Geometry check sheet. Reference: the model listing, model coordinates, mm. A direction names the side the tool comes from. Coordinates: 2 decimals unless noted, no trailing zeros. Write each loop counter-clockwise with the first axis right and the second up, starting at its lowest first coordinate (ties: lowest second). Pieces come first, ordered by that corner, then holes. Notation, with made-up numbers: (-6, 19) -> (13, 19) arc R16 ccw to (13, 41) -> close; hole circle Ø6 at (35, -7). An arc over 180 degrees is marked (long way). Use a Markdown table: item, result.
```python
from build123d import *

# Parameters (mm, degrees)
F1_DEPTH       = 60
F3_D           = 5
F3_CSINK_D     = 7.7
F3_CSINK_ANGLE = 90
F5_DEPTH       = 29.6009997154
F6_W           = 50
F6_H           = 17.8652722283
F7_W           = 50
F7_H           = 17.6054795285
F8_DEPTH       = 5


with BuildPart() as f1:
    # F0 (on Front) → F1 (new body)
    with BuildSketch(Plane.XZ):
        Polygon((-88.3284620883, 15.3996990994), (-88.3284620883, 13.399699384), (-73.3284620883, 13.399699384), (-72.7784620883, 40.999699384), (-13.5784620883, 40.999699384), (-13.0284620883, 13.399699384), (1.9715379117, 13.399699384), (1.9715379117, 15.3996990994), (-11.0679203725, 15.3996990994), (-11.6179203725, 42.9996990994), (-74.7390038042, 42.9996990994), (-75.2890038042, 15.3996990994), align=None)
    extrude(amount=F1_DEPTH)

    # F3 (through all)
    with Locations(Plane.XY.offset(15.3996990994)):
        with Locations((-81.8087329462, -10), (-81.8087329462, -50), (-4.5481912304, -50), (-4.5481912304, -10)):
            CounterSinkHole(F3_D / 2, F3_CSINK_D / 2, counter_sink_angle=F3_CSINK_ANGLE)

    # F4 (on face) → F5 (cut, through all)
    with BuildSketch(Plane.XY.offset(42.9996990994)):
        Polygon((-48.3518556123, -30), (-69.7390038042, -10), (-69.7390038042, -50), align=None)
        Polygon((-21.6179203725, -5), (-64.7390038042, -5), (-43.1784620883, -25.1621474003), align=None)
        Polygon((-16.6179203725, -50), (-16.6179203725, -10), (-38.0050685644, -30), align=None)
        Polygon((-43.1784620883, -34.8378525997), (-64.7390038042, -55), (-21.6179203725, -55), align=None)
    extrude(amount=-F5_DEPTH, mode=Mode.SUBTRACT)

    # F6 (on face) + F7 (on face) → F8 (cut, symmetric)
    with BuildSketch(Plane(origin=(-10.756770725, 0, -0.2143559384), x_dir=(0, 1, 0), z_dir=(0.9998015058, 0, 0.0199235807))):
        with Locations((-30, 29.2899983673)):
            Rectangle(F6_W, F6_H)
    with BuildSketch(Plane(origin=(-75.565874151, 0, 1.505841695), x_dir=(0, -1, 0), z_dir=(-0.9998015058, 0, 0.0199235807))):
        with Locations((30, 27.6993555667)):
            Rectangle(F7_W, F7_H)
    extrude(amount=F8_DEPTH, both=True, dir=(0.9998015058, 0, 0.0199235807), mode=Mode.SUBTRACT)


solid = f1.part
```
Item 1: Depth check by flat-ended pin: P1, Ø6.5, axis at x = -81.81, y = -50, coming from the +Z side; P2, Ø12, axis at y = -12, z = 25, coming from the -X side; P3, Ø1, axis at y = -37, z = 42.5, coming from the -X side. Enter the tip coordinate at first touch or a pass-through.
Answer block:
| item | result |
|---|---|
| P1 | stops at z = 14.8 |
| P2 | stops at x = -75.22 |
| P3 | stops at x = -74.76 |
Item 2: Section check A-A on z = 25. Record the boundary of the cut face in (x, y), then the cut area to 3 significant figures.
Answer block:
| item | result |
|---|---|
| outline | (-75.1, -60) -> (-73.1, -60) -> (-73.1, -55) -> (-75.1, -55) -> close; (-75.1, -5) -> (-73.1, -5) -> (-73.1, 0) -> (-75.1, 0) -> close; (-13.26, -60) -> (-11.26, -60) -> (-11.26, -55) -> (-13.26, -55) -> close; (-13.26, -5) -> (-11.26, -5) -> (-11.26, 0) -> (-13.26, 0) -> close |
| area | 40.0 mm^2 |
Item 3: Tool access check on faces 5 (the flat face through (-32.549, -15.222, 42.014)), 6 (the flat face through (-46.7, -60, 41.4)). Record the directions out of +Z, -Z, +X, -X, +Y, -Y that give a thin tool (end or side, any length) a straight path to the whole face; none if there is none.
Answer block:
| item | result |
|---|---|
| face 5 | +Z, -Z |
| face 6 | +Z, -Z, +X, -X, -Y |
Item 4: Mould release check, pull along Z, two halves, no side actions. Record for faces 1 (the flat face through (-74, -55, 29)), 2 (the flat face through (-6, -30, 13.4)), 3 (the flat face through (-74, -5, 29)), 4 (the flat face through (-27.46, -39.86, 42.01)): +Z half, -Z half, draft (parallel to the pull), parting line (faces both ways), or undercut.
Answer block:
| item | result |
|---|---|
| face 1 | undercut |
| face 2 | -Z half |
| face 3 | undercut |
| face 4 | draft |
Item 5: Thickness scan on L1, parallel to X at y = -10, z = 13.9; L2, parallel to X at y = -4.5, z = 20.75; L3, parallel to Z at x = -12.5, y = -8.5. Record the ranges inside material, lowest first. Write a range as [from, to].
Answer block:
| item | result |
|---|---|
| L1 | x = [-88.33, -84.31], [-79.31, -73.32], [-13.04, -7.05], [-2.05, 1.97] |
| L2 | x = [-75.18, -73.18], [-13.17, -11.17] |
| L3 | z = [13.4, 20.11], [37.98, 43] |
Item 6: Section check B-B on x = -63. Record the boundary of the cut face in (y, z).
Answer block:
| item | result |
|---|---|
| outline | (-60, 41) -> (-55, 41) -> (-55, 43) -> (-60, 43) -> close; (-53.37, 41) -> (-43.7, 41) -> (-43.7, 43) -> (-53.37, 43) -> close; (-16.3, 41) -> (-6.63, 41) -> (-6.63, 43) -> (-16.3, 43) -> close; (-5, 41) -> (0, 41) -> (0, 43) -> (-5, 43) -> close |
Item 7: Section check D-D on y = -20.5. Count the separate pieces of the cut face and the enclosed holes in it, then the cut area to 3 significant figures.
Answer block:
| item | result |
|---|---|
| separate pieces | 6 |
| enclosed holes | 0 |
| area | 153 mm^2 |
Item 8: Section check C-C on z = 17.5. Record the boundary of the cut face in (x, y), then the cut area to 3 significant figures.
Answer block:
| item | result |
|---|---|
| outline | (-75.25, -60) -> (-73.25, -60) -> (-73.25, 0) -> (-75.25, 0) -> close; (-13.11, -60) -> (-11.11, -60) -> (-11.11, 0) -> (-13.11, 0) -> close |
| area | 240 mm^2 |
